For this review, use the dimensioned drawing (mm, ordinates from the lowest corner) and the shaded views. A direction names the side the tool comes from. Round coordinates to 2 decimals unless told otherwise and drop trailing zeros. Order: outer loops, then holes, each group sorted by start corner. A loop starts at its lowest first (then second) coordinate and runs counter-clockwise, first axis right, second up. Notation, with made-up numbers: M -36,46 L -8,46 A5 ccw -8,52 Z; hole C 66.5,73 d10. An arc over 180 degrees is marked long. Answer as CSV lines item,"result". Start each with the question number.
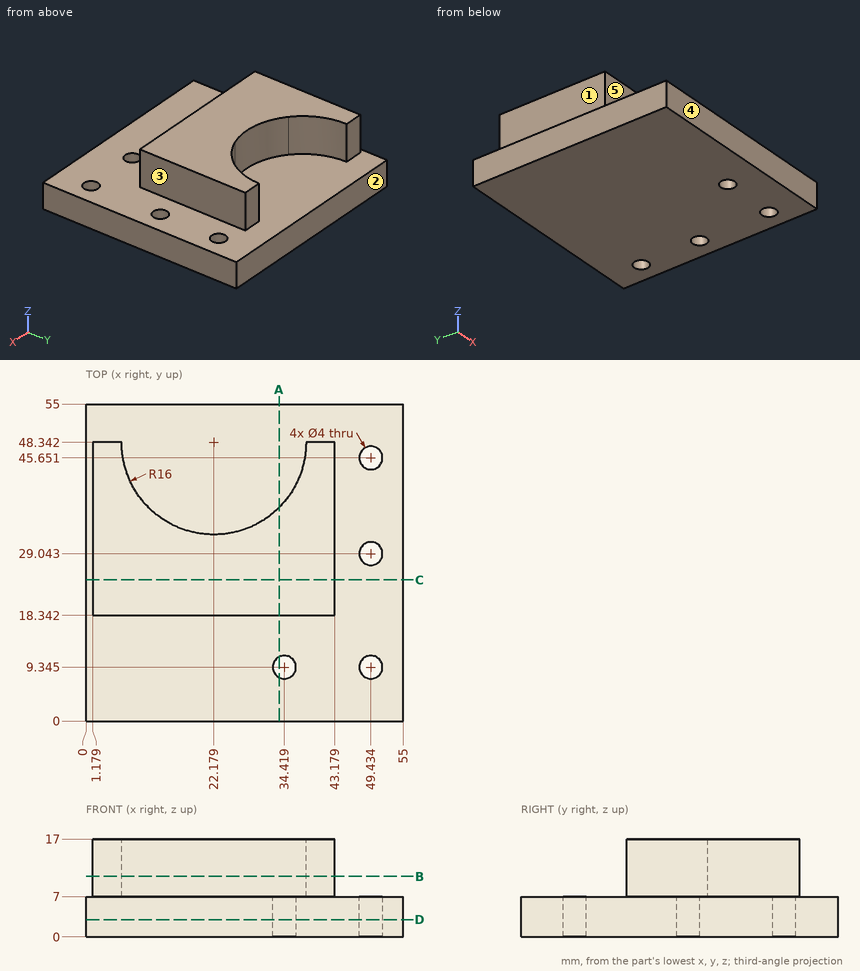
Item 1: Consider section D-D (z = 3). State how many separate pieces and enclosed holes the cut face has.
Item 2: For pin 1 (5.5 mm diameter, centred on x = 41, z = 13.5, fed in from +Y); pin 2 (6 mm diameter, centred on x = 45, y = 39.5, fed in from -Z); pin 3 (2 mm diameter, centred on x = 36.5, y = 44, fed in from +Z); pin 4 (1 mm diameter, centred on x = 25.5, z = 13, fed in from -Y), all flat-tipped, find the tip position at first contact; note any pin that passes through.
Item 3: Tool access review of the marked faces 1, 2, 3, 4 and 5: name each direction out of +Z, -Z, +X, -X, +Y, -Y from which nothing blocks a thin tool from reaching the whole face with its end or side.
Item 4: Consider section C-C (y = 24.5). State the section outline as (x, z) points, and give its area (3 significant figures).
Item 5: Consider section A-A (x = 33.5). State the section outline as (y, z) points, and give its area (3 significant figures).
Item 6: Wall thickness on probe 1 along Z at (x, y) = (27, 14.5); probe 2 along X at (y, z) = (21, 10.75); probe 3 along X at (y, z) = (29.5, 6.5): over which ranges is each line inside the solid? List them lowest first. Write a range as [from, to].
Item 7: Consider section B-B (z = 10.5). State the section outline as (x, y) points, and give its area (3 significant figures).
Reported:
1,separate pieces,"1"
1,enclosed holes,"4"
2,pin 1,"stops at y = 48.34"
2,pin 2,"stops at z = 0"
2,pin 3,"stops at z = 7"
2,pin 4,"stops at y = 18.34"
3,face 1,"+Z, -X, +Y, -Y"
3,face 2,"+Z, -Z, +X, -X, +Y"
3,face 3,"+Z, +X, +Y, -Y"
3,face 4,"+Z, -Z, +X, -X, -Y"
3,face 5,"+Z, +X, -X, -Y"
4,outline,"M 0,0 L 55,0 L 55,7 L 43.18,7 L 43.18,17 L 1.18,17 L 1.18,7 L 0,7 Z"
4,area,"805 mm²"
5,outline,"M 0,0 L 7.57,0 L 7.57,7 L 0,7 Z; M 11.12,0 L 55,0 L 55,7 L 37.04,7 L 37.04,17 L 18.34,17 L 18.34,7 L 11.12,7 Z"
5,area,"547 mm²"
6,probe 1,"z = [0, 7]"
6,probe 2,"x = [1.18, 43.18]"
6,probe 3,"x = [0, 47.49], [51.38, 55]"
7,outline,"M 1.18,18.34 L 43.18,18.34 L 43.18,48.34 L 38.18,48.34 A16 cw 6.18,48.34 L 1.18,48.34 Z"
7,area,"858 mm²"
